```python
from build123d import *

# Parameters (mm, degrees)
F0_W     = 150
F0_H     = 10.3
F1_DEPTH = 6.8
F2_R     = 3.39999
F3_R     = 2.5
F4_DEPTH = 150.001


# Not quite as in the source:
# - a fillet or chamfer is up to 0.001 mm smaller than in the source, because OpenCascade refuses the exact size


with BuildPart() as f1:
    # F0 (on Top) → F1 (new body)
    with BuildSketch(Plane.XY):
        with Locations((47.3209783435, -1.7712331437)):
            Rectangle(F0_W, F0_H)
    extrude(amount=F1_DEPTH)

    # F2 (radius 3.4 in the source; OpenCascade refuses exactly that, so slightly less here)
    f2_edges = [f1.edges().sort_by_distance(p)[0] for p in [
        (47.320978, 3.378767, 6.8),
        (47.320978, 3.378767, 0),
    ]]
    fillet(f2_edges, radius=F2_R)

    # F3 (on face) → F4 (cut, through all)
    with BuildSketch(Plane(origin=(-27.6790216565, 0, 0), x_dir=(0, -1, 0), z_dir=(-1, 0, 0))):
        with Locations((0.0212331437, 3.4)):
            Circle(F3_R)
    extrude(amount=-F4_DEPTH, mode=Mode.SUBTRACT)


solid = f1.part
```
Design review of the part built by this model. Coordinates are the model's own, in mm. Give positions to 0.01 mm unless a question says otherwise; leave off trailing zeros. Write each loop counter-clockwise with the first axis right and the second up, starting at its lowest first coordinate (ties: lowest second). Pieces come first, ordered by that corner, then holes.
(1) Mouldability with a two-part tool opening along Y and no side actions: class faces 1 (the face through (46.27, 0.3, 5.88)), 2 (the face through (48.371, 2.409, 1.022)), 3 (the face through (-27.679, -3, 3)) as +Y half, -Y half, draft (parallel to the pull), parting line (faces both ways), or undercut.
Checked values:
face 1: undercut
face 2: +Y half
face 3: draft
(2) Wall thickness on line 1 along Z through (x, y) = (50.5, 0.25); line 2 along Z through (x, y) = (22.5, 1.25); line 3 along Y through (x, z) = (54, 4): over which ranges is each line inside the solid? List them lowest first.
Checked values:
line 1: z = 0.01 to 0.91, 5.89 to 6.79
line 2: z = 0.25 to 1.25, 5.55 to 6.55
line 3: y = -6.92 to -2.45, 2.41 to 3.33
(3) Clearance check with flat-ended pins moving along their axes: pin 1 Ø4 at (y, z) = (0, 3) entering from +X; pin 2 Ø4 at (y, z) = (0.5, 5.5) entering from -X. State where each tip first meets the part, or that it passes through.
Checked values:
pin 1: passes through
pin 2: stops at x = -27.68
(4) Add section A-A (y = -1.25). Give the boundary of the cut face in (x, z), and give its area (3 significant figures).
Checked values:
outline: (-27.68, 0) - (122.32, 0) - (122.32, 1.22) - (-27.68, 1.22) - close; (-27.68, 5.58) - (122.32, 5.58) - (122.32, 6.8) - (-27.68, 6.8) - close
area: 367 mm2
